from build123d import *

# Parameters (mm, degrees)
F0_R     = 2
F1_DEPTH = 20
F2_R     = 4.7152449582
F2_R_2   = 4.7232891339
F3_DEPTH = 108
F4_R     = 4.2098088582
F5_DEPTH = 25
F6_R     = 3.1711780618
F6_R_2   = 3.2066806009
F6_R_3   = 3.1312270379
F6_W     = 0.6074849516
F6_H     = 3.2243365422
F6_W_2   = 0.6542131305
F7_DEPTH = 25


# Not quite as in the source:
# - a feature names something its author has since deleted; it is built from what else it names


with BuildPart() as f1:
    # F0 (on Top) → F1 (new body)
    with BuildSketch(Plane.XY):
        with BuildLine():
            Line((-164.65269916, 33.20941329), (-164.65269916, 32.9194632454))
            ThreePointArc((-164.65269916, 32.9194632454), (-165.5739976736, 29.1538786951), (-166.563206189, 32.902196247))
            Line((-166.563206189, 32.902196247), (-166.563206189, 33.20941329))
            Line((-166.563206189, 33.20941329), (-170, 33.20941329))
            Line((-170, 33.20941329), (-170, 0))
            Line((-170, 0), (-170, -33.20941329))
            Line((-170, -33.20941329), (-166.563206189, -33.20941329))
            Line((-166.563206189, -33.20941329), (-166.563206189, -32.902196247))
            ThreePointArc((-166.563206189, -32.902196247), (-165.5739976736, -29.1538786951), (-164.65269916, -32.9194632454))
            Line((-164.65269916, -32.9194632454), (-164.65269916, -33.20941329))
            Line((-164.65269916, -33.20941329), (-163.2265451578, -33.20941329))
            Line((-163.2265451578, -33.20941329), (-159.009280774, -33.20941329))
            Line((-159.009280774, -33.20941329), (-159.009280774, -36.7204154693))
            Line((-159.009280774, -36.7204154693), (-157.7970415085, -36.7204154693))
            Line((-157.7970415085, -36.7204154693), (-128.8103089121, -36.7204154693))
            ThreePointArc((-128.8103089121, -36.7204154693), (-115.3036395578, -25.0214683637), (-99.1359348061, -32.6307261124))
            ThreePointArc((-99.1359348061, -32.6307261124), (-97.3177205123, -34.3677013727), (-94.8839611325, -35))
            Line((-94.8839611325, -35), (-6.3253850676, -35))
            ThreePointArc((-6.3253850676, -35), (-4.9357568901, -37.0403297798), (-2.4707801799, -37.1741277646))
            Line((-2.4707801799, -37.1741277646), (0, -38.1401939384))
            Line((0, -38.1401939384), (0, -35))
            Line((0, -35), (0, 0))
            Line((0, 0), (0, 35))
            Line((0, 35), (0, 38.1401939384))
            Line((0, 38.1401939384), (-2.4707801799, 37.1741277646))
            ThreePointArc((-2.4707801799, 37.1741277646), (-4.9357568901, 37.0403297798), (-6.3253850676, 35))
            Line((-6.3253850676, 35), (-94.8839611325, 35))
            ThreePointArc((-94.8839611325, 35), (-97.3177205123, 34.3677013727), (-99.1359348061, 32.6307261124))
            ThreePointArc((-99.1359348061, 32.6307261124), (-115.3036395578, 25.0214683637), (-128.8103089121, 36.7204154693))
            Line((-128.8103089121, 36.7204154693), (-157.7970415085, 36.7204154693))
            Line((-157.7970415085, 36.7204154693), (-159.009280774, 36.7204154693))
            Line((-159.009280774, 36.7204154693), (-159.009280774, 33.20941329))
            Line((-159.009280774, 33.20941329), (-163.2265451578, 33.20941329))
            Line((-163.2265451578, 33.20941329), (-164.65269916, 33.20941329))
        make_face()
        with Locations((-94.8839611325, -30)):
            Circle(F0_R, mode=Mode.SUBTRACT)
        with BuildLine():
            ThreePointArc((-1.5680128924, -34.6153974533), (-1.5847981725, -34.8739692511), (-1.6348722671, -35.1282008489))
            ThreePointArc((-1.6348722671, -35.1282008489), (-3.5680128924, -36.6153974533), (-5.5011535178, -35.1282008489))
            ThreePointArc((-5.5011535178, -35.1282008489), (-5.561565475, -34.4549353061), (-5.3942458987, -33.8))
            ThreePointArc((-5.3942458987, -33.8), (-3.5680128924, -32.6153974533), (-1.7417798862, -33.8))
            ThreePointArc((-1.7417798862, -33.8), (-1.6119369721, -34.1985437695), (-1.5680128924, -34.6153974533))
        make_face(mode=Mode.SUBTRACT)
        with Locations((-94.8839611325, 30)):
            Circle(F0_R, mode=Mode.SUBTRACT)
        with BuildLine():
            Line((-1.5434729926, 32.5735324938), (-1.2, 32.5194895267))
            Line((-1.2, 32.5194895267), (-1.2, 0))
            Line((-1.2, 0), (-1.2, -32.5194895267))
            Line((-1.2, -32.5194895267), (-1.5434729926, -32.5735324938))
            ThreePointArc((-1.5434729926, -32.5735324938), (-4.2823772406, -31.8301402125), (-6.3253850676, -33.8))
            Line((-6.3253850676, -33.8), (-90.2593984932, -33.8))
            Line((-90.2593984932, -33.8), (-92.2271985619, -31.6787384118))
            ThreePointArc((-92.2271985619, -31.6787384118), (-92.912700117, -27.5524134293), (-97.0903228742, -27.7620281778))
            Line((-97.0903228742, -27.7620281778), (-101.4582490544, -28.045448372))
            ThreePointArc((-101.4582490544, -28.045448372), (-117.5672901619, -24.2537650751), (-129.6891982841, -35.5204154693))
            Line((-129.6891982841, -35.5204154693), (-155.884909603, -35.5204154693))
            Line((-155.884909603, -35.5204154693), (-157.7970415085, -35.5204154693))
            Line((-157.7970415085, -35.5204154693), (-157.7970415085, -32.2268303811))
            Line((-157.7970415085, -32.2268303811), (-162.8932879486, -32.2268303811))
            ThreePointArc((-162.8932879486, -32.2268303811), (-163.6774302758, -28.9699966079), (-167.0088434251, -28.6185256358))
            Line((-167.0088434251, -28.6185256358), (-167.2241950518, -28.4767444108))
            Line((-167.2241950518, -28.4767444108), (-168.8, -27.1884445101))
            Line((-168.8, -27.1884445101), (-168.8, 0))
            Line((-168.8, 0), (-168.8, 27.1884445101))
            Line((-168.8, 27.1884445101), (-167.2241950518, 28.4767444108))
            Line((-167.2241950518, 28.4767444108), (-167.0088434251, 28.6185256358))
            ThreePointArc((-167.0088434251, 28.6185256358), (-163.6774302758, 28.9699966079), (-162.8932879486, 32.2268303811))
            Line((-162.8932879486, 32.2268303811), (-157.7970415085, 32.2268303811))
            Line((-157.7970415085, 32.2268303811), (-157.7970415085, 35.5204154693))
            Line((-157.7970415085, 35.5204154693), (-155.884909603, 35.5204154693))
            Line((-155.884909603, 35.5204154693), (-129.6891982841, 35.5204154693))
            ThreePointArc((-129.6891982841, 35.5204154693), (-117.5672901619, 24.2537650751), (-101.4582490544, 28.045448372))
            Line((-101.4582490544, 28.045448372), (-97.0903228742, 27.7620281778))
            ThreePointArc((-97.0903228742, 27.7620281778), (-92.912700117, 27.5524134293), (-92.2271985619, 31.6787384118))
            Line((-92.2271985619, 31.6787384118), (-90.2593984932, 33.8))
            Line((-90.2593984932, 33.8), (-6.3253850676, 33.8))
            ThreePointArc((-6.3253850676, 33.8), (-4.2823772406, 31.8301402125), (-1.5434729926, 32.5735324938))
        make_face(mode=Mode.SUBTRACT)
        with BuildLine():
            ThreePointArc((-1.7417798862, 33.8), (-3.5680128924, 32.6153974533), (-5.3942458987, 33.8))
            ThreePointArc((-5.3942458987, 33.8), (-5.561565475, 34.4549353061), (-5.5011535178, 35.1282008489))
            ThreePointArc((-5.5011535178, 35.1282008489), (-3.5680128924, 36.6153974533), (-1.6348722671, 35.1282008489))
            ThreePointArc((-1.6348722671, 35.1282008489), (-1.5847981725, 34.8739692511), (-1.5680128924, 34.6153974533))
            ThreePointArc((-1.5680128924, 34.6153974533), (-1.6119369721, 34.1985437695), (-1.7417798862, 33.8))
        make_face(mode=Mode.SUBTRACT)
    extrude(amount=F1_DEPTH)

    # F2 (on face) → F3 (cut)
    with BuildSketch(Plane.XZ.offset(36.7204154693)):
        with Locations((-149.9848365784, 9.8437862471)):
            Circle(F2_R)
        with Locations((-17.5157543272, 9.6355015412)):
            Circle(F2_R_2)
    extrude(amount=-F3_DEPTH, mode=Mode.SUBTRACT)

    # F4 (on face) → F5 (cut)
    with BuildSketch(Plane(origin=(-170, 0, 0), x_dir=(0, -1, 0), z_dir=(-1, 0, 0))):
        with Locations((0, 10.2570122108)):
            Circle(F4_R)
    extrude(amount=-F5_DEPTH, mode=Mode.SUBTRACT)

    # F6 (on face) → F7 (cut)
    with BuildSketch(Plane.YZ):
        with Locations((0, 3.6681490019)):
            Circle(F6_R)
        with Locations((16.0749554634, 3.6681490019)):
            Circle(F6_R_2)
        with Locations((-18.6450798064, 3.6681490019)):
            Circle(F6_R_3)
        with Locations((-21.4254865423, 12.4766645022)):
            Rectangle(F6_W, F6_H)
        with Locations((-16.1684155464, 12.4766645022)):
            Rectangle(F6_W_2, F6_H)
    extrude(amount=-F7_DEPTH, mode=Mode.SUBTRACT)


solid = f1.part
Source: CAD feature listing. Evaluate the final solid. Frame: model axes, mm. A direction names the side the tool comes from. Round coordinates to 2 decimals unless told otherwise and drop trailing zeros. Loops run counter-clockwise (first coordinate to the right, second up) from the corner with the lowest first, then second, coordinate; pieces in that order, holes last. Notation, with made-up numbers: M -10,25 L 29,25 A24 cw 29,45 Z; hole C 77,70.5 d3. An arc over 180 degrees is marked long. Return JSON: item names as keys, results as strings. Group by question number.
1. Section query D-D on z = 17.5. State how many separate pieces and enclosed holes the cut face has, and give its area (3 significant figures).
2. Section query A-A on y = 8.5. Output: boundary loops of the cut face in (x, z).
3. Mould query, pull axis X, two halves, no side actions, for faces 1 (the face through (0, -1, 10)), 2 (the face through (-13.01, -34.41, 11.05)), 3 (the face through (-144, 36.72, 10)). Classes: released by +X, released by -X, zero draft, split by the parting line, or undercut.
4. Section query B-B on x = -32. Output: boundary loops of the cut face in (y, z), and give its area (3 significant figures).
5. Pin query (flat end, axial travel): pin 1 (1 mm diameter, centred on x = -121, z = 14.5, fed in from -Y); pin 2 (1.5 mm diameter, centred on x = -17.5, z = 5.5, fed in from -Y); pin 3 (5.5 mm diameter, centred on x = -149.98, z = 9.84, fed in from +Y); pin 4 (0.6 mm diameter, centred on x = -0.5, z = 13, fed in from -Y). Return the tip coordinate at first contact, or that it passes through.
6. Section query C-C on y = 0. Output: boundary loops of the cut face in (x, z), and give its area (3 significant figures).
7. Reachability of faces 4 (the face through (-4.24, -31.82, 9.86)), 5 (the face through (-0.59, -15.66, 4.61)), 6 (the face through (-144, -36.72, 10)), 7 (the face through (-115.041, 24.987, 9.86)), 8 (the face through (-159.009, 35, 10)) from +Z, -Z, +X, -X, +Y, -Y: full face, straight path, thin tool, end or side. Return the list, or none.
8. Material intervals for line 1 along Y through (x, z) = (-137.5, 4); line 2 along Y through (x, z) = (-33, 17); line 3 along X through (y, z) = (-5.5, 8.75), sorted ascending. Write a range as from..to.
Checks:
{
 "1": {"separate pieces": "1", "enclosed holes": "5", "area": "697 mm²"},
 "2": {"outline": "M -170,0 L -168.8,0 L -168.8,20 L -170,20 Z; M -1.2,0 L 0,0 L 0,20 L -1.2,20 Z"},
 "3": {"face 1": "released by +X", "face 2": "undercut", "face 3": "zero draft"},
 "4": {"outline": "M -35,0 L -33.8,0 L -33.8,20 L -35,20 Z; M 33.8,0 L 35,0 L 35,20 L 33.8,20 Z", "area": "48.0 mm²"},
 "5": {"pin 1": "stops at y = -27.21", "pin 2": "stops at y = -35", "pin 3": "passes through", "pin 4": "stops at y = -38.06"},
 "6": {"outline": "M -170,0 L -168.8,0 L -168.8,6.05 L -170,6.05 Z; M -170,14.47 L -168.8,14.47 L -168.8,20 L -170,20 Z; M -1.2,0 L 0,0 L 0,0.5 L -1.2,0.5 Z; M -1.2,6.84 L 0,6.84 L 0,20 L -1.2,20 Z", "area": "30.3 mm²"},
 "7": {"face 4": "+Z, -Z", "face 5": "+X", "face 6": "+Z, -Z, -X, -Y", "face 7": "+Z, -Z, +Y", "face 8": "+Z, -Z, -X, +Y"},
 "8": {"line 1": "y = -36.72..-35.52, 35.52..36.72", "line 2": "y = -35..-33.8, 33.8..35", "line 3": "x = -170..-168.8, -1.2..0"}
}
